Verification items for this drawing (mm, ordinates from the low corner). Give positions to 0.01 mm unless a question says otherwise; leave off trailing zeros. Write each loop counter-clockwise with the first axis right and the second up, starting at its lowest first coordinate (ties: lowest second). Pieces come first, ordered by that corner, then holes. Notation, with made-up numbers: M 41.25,-4.5 L 96.25,-4.5 A24 ccw 96.25,18.5 Z; hole C 3,27.25 d11. An arc over 180 degrees is marked long. Use one line per item in the form item = value. Start each with the question number.
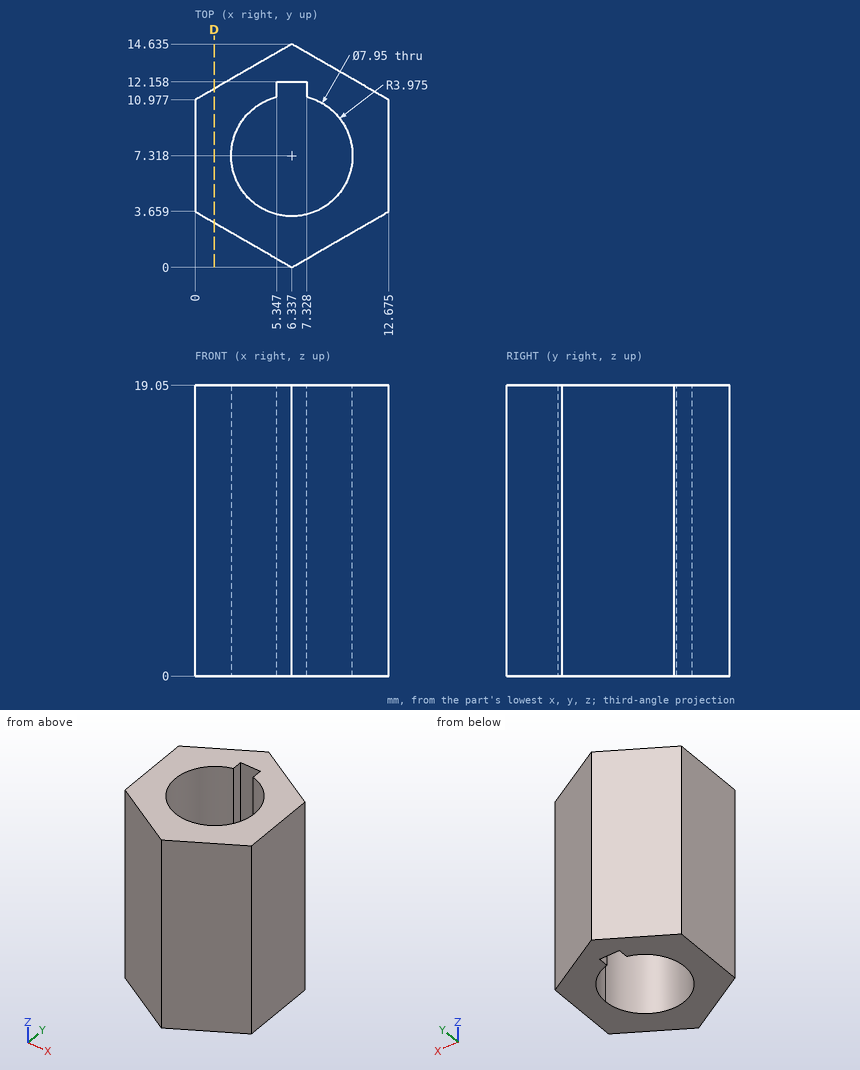
(1) Sectioned sample at D-D, the plane x = 1.25. Record the boundary of the cut face in (y, z), plus the area to 3 significant figures.
(2) Thickness scan on probe 1 along Y at (x, z) = (10, 14.5) (1 decimal); probe 2 along Y at (x, z) = (4.5, 18) (1 decimal); probe 3 along X at (y, z) = (4.5, 6.25) (1 decimal). Record the ranges inside material, lowest first. Write a range as [from, to].
(3) Depth check by flat-ended pin: pin 1 (1.5 mm diameter, centred on x = 5, y = 6, fed in from +Z); pin 2 (0.5 mm diameter, centred on y = 11.5, z = 12, fed in from +X); pin 3 (2 mm diameter, centred on x = 6, z = 10, fed in from -Y); pin 4 (0.8 mm diameter, centred on y = 11.5, z = 12.5, fed in from -X) (1 decimal). Enter the tip coordinate at first touch or a pass-through.
Numbers:
q1.outline = M 2.94,0 L 11.7,0 L 11.7,19.05 L 2.94,19.05 Z
q1.area = 167 mm2
q2.probe_1 = [2.1, 5.8], [8.9, 12.5]
q2.probe_2 = [1.1, 3.8], [10.8, 13.6]
q2.probe_3 = [0, 3.5], [9.1, 12.7]
q3.pin_1 = through
q3.pin_2 = 12.2
q3.pin_3 = 0
q3.pin_4 = 0.2
